```python
from build123d import *

# Parameters (mm, degrees)
CYLINDER003_R      = 25.4
CYLINDER003_DEPTH  = 3.17
CYLINDER001_R      = 12.7
CYLINDER001_DEPTH  = 50.8
CYLINDER004_R      = 25.4
CYLINDER004_DEPTH  = 3.17
FUSION_PITCH_ANGLE = 90


with BuildPart() as cylinder003:
    # Cylinder003 → Cylinder003 (new body)
    with BuildSketch(Plane.XY):
        Circle(CYLINDER003_R)
    extrude(amount=CYLINDER003_DEPTH)


with BuildPart() as cylinder001:
    # Cylinder001 → Cylinder001 (new body)
    with BuildSketch(Plane.XY):
        Circle(CYLINDER001_R)
    extrude(amount=CYLINDER001_DEPTH)


with BuildPart() as fusion:
    # Cylinder004 → Cylinder004 (new body)
    with BuildSketch(Plane.XY.offset(50.8)):
        Circle(CYLINDER004_R)
    extrude(amount=CYLINDER004_DEPTH)

    # Fusion: union Cylinder003, Cylinder001
    add(cylinder003.part)
    add(cylinder001.part)


with BuildPart() as fusion_1:
    # Fusion pitch: moved
    add(fusion.part.rotate(Axis((0, 0, 0), (0, 1, 0)), FUSION_PITCH_ANGLE))


with BuildPart() as fusion_2:
    # Fusion placement: moved
    add(fusion_1.part.moved(Location((-22.347, 11.43, 50.8))))


solid = fusion_2.part
```
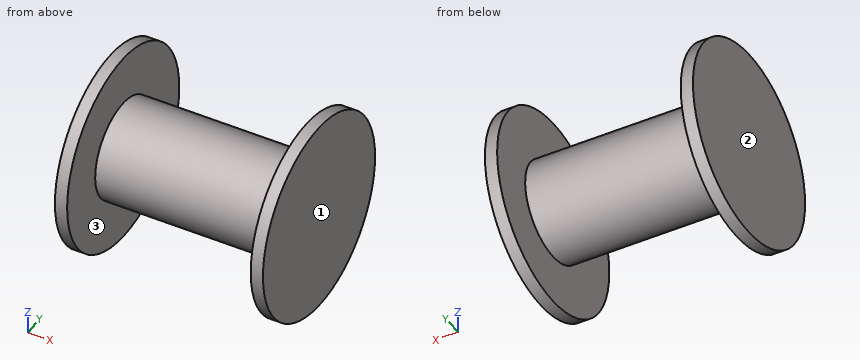
Input: part model. Units: mm. Frame: model coordinates. Face numbers are marked on the shaded views. Coordinates: 2 decimals unless noted, no trailing zeros. Write each loop counter-clockwise with the first axis right and the second up, starting at its lowest first coordinate (ties: lowest second). Pieces come first, ordered by that corner, then holes. Notation, with made-up numbers: M 58.25,62 L 75.25,62 A17 cw 75.25,70 Z; hole C 58,-6 d8. An arc over 180 degrees is marked long. Use one line per item in the form item = value.
Q1. Material intervals for probe 1 along X at (y, z) = (-6.5, 34); probe 2 along Z at (x, y) = (16, 18); probe 3 along Y at (x, z) = (-17.5, 56), sorted ascending. Write a range as from..to.
Answer below:
probe_1 = -22.35..-19.18, 28.45..31.62
probe_2 = 39.93..61.67
probe_3 = -0.16..23.02
Q2. Section A-A (y = 11.43). Return loops of the section in (x, z), plus the area to 3 significant figures.
Answer below:
outline = M -22.35,25.4 L -19.18,25.4 L -19.18,38.1 L 28.45,38.1 L 28.45,25.4 L 31.62,25.4 L 31.62,76.2 L 28.45,76.2 L 28.45,63.5 L -19.18,63.5 L -19.18,76.2 L -22.35,76.2 Z
area = 1,530 mm²
Q3. Section C-C (y = -2). Return loops of the section in (x, z), plus the area to 3 significant figures.
Answer below:
outline = M -22.35,29.24 L -19.18,29.24 L -19.18,72.36 L -22.35,72.36 Z; M 28.45,29.24 L 31.62,29.24 L 31.62,72.36 L 28.45,72.36 Z
area = 273 mm²
Q4. First-contact query: pin 1 (6 mm diameter, centred on x = 17.5, z = 49.5, fed in from -Y); pin 2 (12 mm diameter, centred on x = -3, y = -3, fed in from -Z); pin 3 (2 mm diameter, centred on x = 18.5, y = 23, fed in from -Z). Flat tips, straight axial feed; report the tip coordinate or a pass-through.
Answer below:
pin_1 = -1.27
pin_2 = 41.3
pin_3 = 43.76
Q5. Section B-B (z = 69.5). Return loops of the section in (x, y).
Answer below:
outline = M -22.35,-5.76 L -19.18,-5.76 L -19.18,28.62 L -22.35,28.62 Z; M 28.45,-5.76 L 31.62,-5.76 L 31.62,28.62 L 28.45,28.62 Z
Q6. Draft query along X for the marked faces 1, 2 and 3. Return one class per face: released by +X, released by -X, zero draft, split by the parting line, or undercut.
Answer below:
face_1 = released by +X
face_2 = released by -X
face_3 = undercut
Q7. Section D-D (x = 16). Return loops of the section in (y, z), plus the area to 3 significant figures.
Answer below:
outline = C 11.43,50.8 d25.4
area = 507 mm²
